Source: CAD feature listing. Evaluate the final solid. Frame: model axes, mm. Face numbers are marked on the shaded views. A direction names the side the tool comes from. Round coordinates to 2 decimals unless told otherwise and drop trailing zeros. Write each loop counter-clockwise with the first axis right and the second up, starting at its lowest first coordinate (ties: lowest second). Pieces come first, ordered by that corner, then holes.
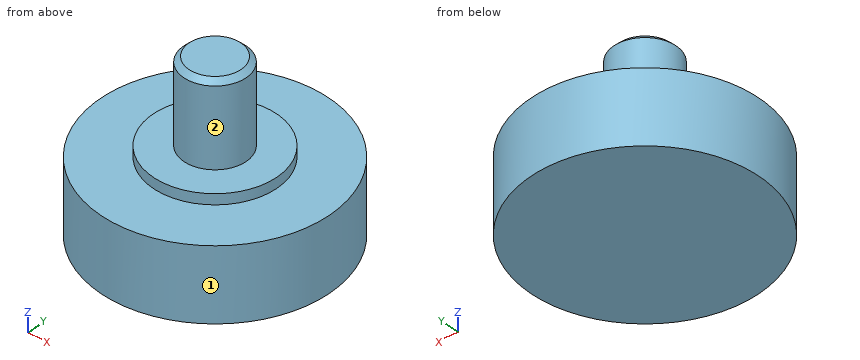
Autodesk Inventor part; units mm, degrees
ref_plane "YZ Plane" through (0, 0, 0) normal (1, 0, 0) x (0, 1, 0)
ref_plane "XZ Plane" through (0, 0, 0) normal (0, 1, 0) x (-1, 0, 0)
ref_plane "XY Plane" through (0, 0, 0) normal (0, 0, 1) x (1, 0, 0)
sketch "草圖1" plane through (0, 0, 0) normal (0, 0, 1) x (1, 0, 0)
  circle A0 centre (0, 0) radius 11
  dimension "d0" = 22
extrude "擠出1" add sketch "草圖1" along normal blind 7
sketch "草圖2" plane through (0, 0, 7) normal (0, 0, 1) x (1, 0, 0)
  circle A0 centre (0, 0) radius 5.95
  dimension "d3" = 11.9
extrude "擠出2" add sketch "草圖2" along normal blind 1
sketch "草圖3" plane through (0, 0, 8) normal (0, 0, 1) x (1, 0, 0)
  circle A0 centre (0, 0) radius 3
  dimension "d6" = 6
extrude "擠出3" add sketch "草圖3" along normal blind 8
chamfer "倒角1" distance 0.5 angle 45 1 edges at (-3, 0, 16)
properties part number "bearing 22-M6"
1) Reachability of the marked faces 1 and 2 from +Z, -Z, +X, -X, +Y, -Y: full face, straight path, thin tool, end or side. Return the list, or none.
Taken from the geometry:
face 1: +Z, -Z
face 2: +Z
2) Section query A-A on x = 0. Return the cut outline in (y, z), then the cut area to 3 significant figures.
Taken from the geometry:
outline: (-11, 0) - (11, 0) - (11, 7) - (5.95, 7) - (5.95, 8) - (3, 8) - (3, 15.5) - (2.5, 16) - (-2.5, 16) - (-3, 15.5) - (-3, 8) - (-5.95, 8) - (-5.95, 7) - (-11, 7) - close
area: 214 mm2
3) Section query C-C on z = 9. Return the cut outline in (x, y).
Taken from the geometry:
outline: circle Ø6 at (0, 0)
4) Section query D-D on x = 5.25. Return the cut outline in (y, z).
Taken from the geometry:
outline: (-9.67, 0) - (9.67, 0) - (9.67, 7) - (2.8, 7) - (2.8, 8) - (-2.8, 8) - (-2.8, 7) - (-9.67, 7) - close
5) Material intervals for line 1 (Z direction, x = 4.75, y = -9); line 2 (Y direction, x = 0, z = 7.25); line 3 (Z direction, x = 5, y = 2), sorted ascending.
Taken from the geometry:
line 1: z = 0 to 7
line 2: y = -5.95 to 5.95
line 3: z = 0 to 8
6) Contact query for flat-ended pins moving along their axis: P1, Ø6, axis at x = -7.5, z = 12.5, coming from the -Y side; P2, Ø6, axis at y = -5, z = 2.5, coming from the +X side; P3, Ø12, axis at x = 6, y = 6.5, coming from the +Z side; P4, Ø6, axis at x = -8.5, z = 3, coming from the +Y side. Output: stop coordinate, or through.
Taken from the geometry:
P1: passes through
P2: stops at x = 10.82
P3: stops at z = 15.65
P4: stops at y = 9.53
